The drawing under review shows one solid part. Ordinate dimensions are in mm from its lowest x, y, z. Coordinates: 2 decimals unless noted, no trailing zeros. Write each loop counter-clockwise with the first axis right and the second up, starting at its lowest first coordinate (ties: lowest second). Pieces come first, ordered by that corner, then holes.
Q1. Clearance check with flat-ended pins moving along their axes: pin 1 Ø3.5 at (x, y) = (12.7, 29.21) entering from -Z; pin 2 Ø1 at (x, z) = (2.5, 0.5) entering from +Y (1 decimal). State where each tip first meets the part, or that it passes through.
Q2. Add section A-A, the plane x = 12.7. Give the boundary of the cut face in (y, z) (1 decimal).
Q3. Add section C-C, the plane y = 29.21. Give the boundary of the cut face in (x, z) (1 decimal).
Q4. To check wall thickness, follow probe 1 along Y at (x, z) = (12.7, 0.95) (1 decimal); probe 2 along X at (y, z) = (63.5, 2.2) (1 decimal); probe 3 along Y at (x, z) = (12, 2.3) (1 decimal). State the ranges of each line that lie inside material, in increasing order.
Q5. Add section D-D, the plane y = 70.5. Give the boundary of the cut face in (x, z) (1 decimal).
Q6. Add section B-B, the plane z = 2.4. Give the boundary of the cut face in (x, y) (1 decimal), plus the area to 3 significant figures.
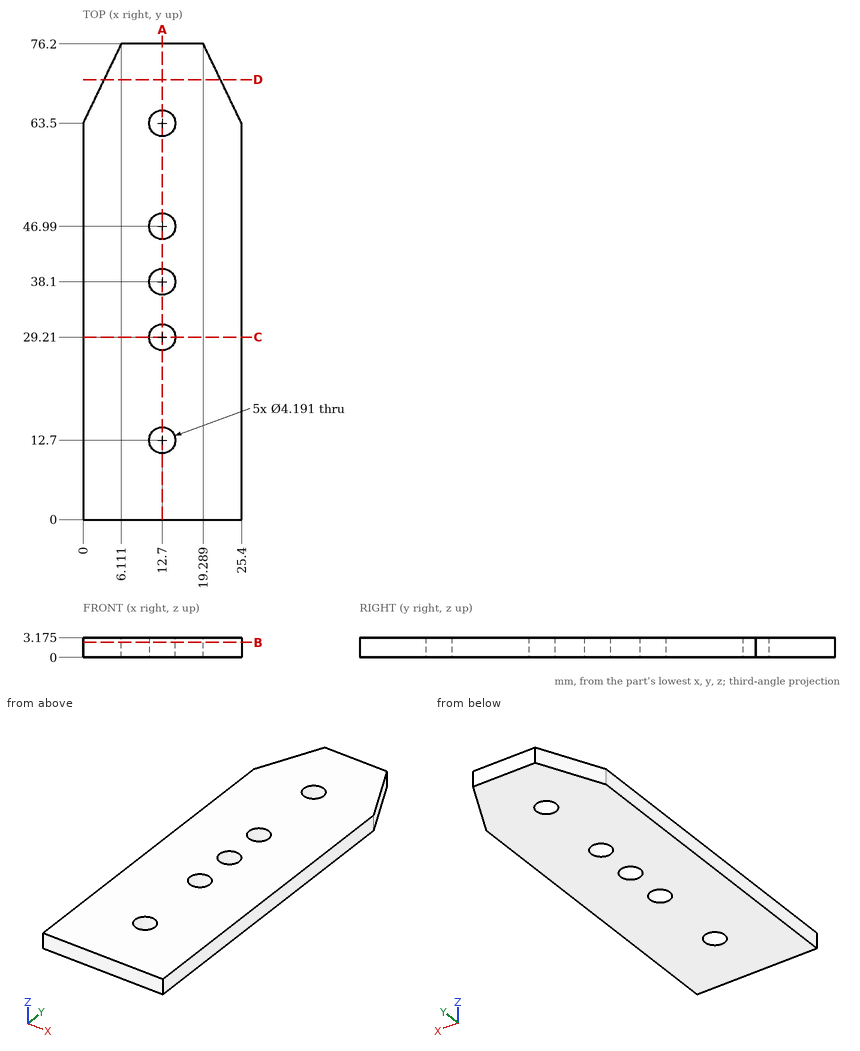
Here are the results:
1. pin 1: passes through
1. pin 2: stops at y = 69.7
2. outline: (0, 0) - (10.6, 0) - (10.6, 3.2) - (0, 3.2) - close; (14.8, 0) - (27.1, 0) - (27.1, 3.2) - (14.8, 3.2) - close; (31.3, 0) - (36, 0) - (36, 3.2) - (31.3, 3.2) - close; (40.2, 0) - (44.9, 0) - (44.9, 3.2) - (40.2, 3.2) - close; (49.1, 0) - (61.4, 0) - (61.4, 3.2) - (49.1, 3.2) - close; (65.6, 0) - (76.2, 0) - (76.2, 3.2) - (65.6, 3.2) - close
3. outline: (0, 0) - (10.6, 0) - (10.6, 3.2) - (0, 3.2) - close; (14.8, 0) - (25.4, 0) - (25.4, 3.2) - (14.8, 3.2) - close
4. probe 1: y = 0 to 10.6, 14.8 to 27.1, 31.3 to 36, 40.2 to 44.9, 49.1 to 61.4, 65.6 to 76.2
4. probe 2: x = 0 to 10.6, 14.8 to 25.4
4. probe 3: y = 0 to 10.7, 14.7 to 27.2, 31.2 to 36.1, 40.1 to 45, 49 to 61.5, 65.5 to 76.2
5. outline: (3.4, 0) - (22, 0) - (22, 3.2) - (3.4, 3.2) - close
6. outline: (0, 0) - (25.4, 0) - (25.4, 63.5) - (19.3, 76.2) - (6.1, 76.2) - (0, 63.5) - close; hole circle Ø4.2 at (12.7, 12.7); hole circle Ø4.2 at (12.7, 29.2); hole circle Ø4.2 at (12.7, 38.1); hole circle Ø4.2 at (12.7, 47); hole circle Ø4.2 at (12.7, 63.5)
6. area: 1,790 mm2
